```python
from build123d import *

# Parameters (mm, degrees)
SKETCH1_W           = 30
SKETCH1_H           = 120
BOSS_EXTRUDE1_DEPTH = 39
SKETCH2_OUTSIDE_W   = 57.94
SKETCH2_OUTSIDE_H   = 147.94
CUT_EXTRUDE2_DEPTH  = 74.116345642
FILLET1_R           = 5
CUT_EXTRUDE3_DEPTH  = 74.116345642
SKETCH4_W           = 4
SKETCH4_H           = 90
CUT_EXTRUDE4_DEPTH  = 72.902712049
SKETCH5_R           = 2
CUT_EXTRUDE5_DEPTH  = 72.902712049


with BuildPart() as part:
    # Sketch1 → Boss-Extrude1 (new body)
    with BuildSketch(Plane(origin=(0, 0, 0), x_dir=(1, 0, 0), z_dir=(0, 1, 0))):
        Rectangle(SKETCH1_W, SKETCH1_H)
    extrude(amount=BOSS_EXTRUDE1_DEPTH)

    # Sketch2 outside → Cut-Extrude2 (cut, through all)
    with BuildSketch(Plane(origin=(0, 39, 0), x_dir=(1, 0, 0), z_dir=(0, 1, 0))):
        Rectangle(SKETCH2_OUTSIDE_W, SKETCH2_OUTSIDE_H)
        Polygon((0, 60), (-15, 34.019237886), (-15, -60), (15, -60), (15, 34.019237886), align=None, mode=Mode.SUBTRACT)
    extrude(amount=-CUT_EXTRUDE2_DEPTH, mode=Mode.SUBTRACT)

    # Fillet1
    fillet1_edges = [part.edges().sort_by_distance(p)[0] for p in [
        (0, 19.5, -60),
    ]]
    fillet(fillet1_edges, radius=FILLET1_R)

    # Sketch3 → Cut-Extrude3 (cut, through all)
    with BuildSketch(Plane(origin=(0, 39, 0), x_dir=(1, 0, 0), z_dir=(0, 1, 0))):
        Polygon((-15, 34.019237886), (-15, -60), (-7, -60), (-7, 47.875644347), align=None)
        Polygon((7, 47.875644347), (7, -60), (15, -60), (15, 34.019237886), align=None)
    extrude(amount=-CUT_EXTRUDE3_DEPTH, mode=Mode.SUBTRACT)

    # Sketch4 → Cut-Extrude4 (cut, through all)
    with BuildSketch(Plane(origin=(0, 39, 0), x_dir=(1, 0, 0), z_dir=(0, 1, 0))):
        with Locations((-5, -15)):
            Rectangle(SKETCH4_W, SKETCH4_H)
    extrude(amount=-CUT_EXTRUDE4_DEPTH, mode=Mode.SUBTRACT)

    # Sketch5 → Cut-Extrude5 (cut, through all)
    with BuildSketch(Plane(origin=(0, 39, 0), x_dir=(1, 0, 0), z_dir=(0, 1, 0))):
        with Locations(Location((0, 46, 0), (0, 0, 270))):
            Circle(SKETCH5_R)
    extrude(amount=-CUT_EXTRUDE5_DEPTH, mode=Mode.SUBTRACT)


solid = part.part
```
Read the model definition and answer for the solid it produces. Units are mm, in the model's axes. A direction names the side the tool comes from. Coordinates: 2 decimals unless noted, no trailing zeros. Order: outer loops, then holes, each group sorted by start corner. A loop starts at its lowest first (then second) coordinate and runs counter-clockwise, first axis right, second up. Notation, with made-up numbers: (16.5, -1) - (68.5, -1) arc R29 ccw to (68.5, 29) - close; hole circle Ø7 at (69.25, -32). An arc over 180 degrees is marked (long way). Answer as a JSON object with one key per item and string values. Group by question number.
Item 1: Section C-C (z = 20) is taken. Give the vertices of the cut face in (x, y), plus the area to 3 significant figures.
Item 2: Section D-D (x = 6) is taken. Give the vertices of the cut face in (y, z), plus the area to 3 significant figures.
Item 3: The mould has two halves that part along Z. Classify faces 1 (the face through (-7, 20, -39)), 2 (the face through (5.68, 19.77, -50.16)), 3 (the face through (0, 20, -48)), 4 (the face through (2, 19, 60)): +Z half, -Z half, draft (parallel to the pull), parting line (faces both ways), or undercut.
Item 4: Flat-ended cylindrical pins translate along their axes: P1, Ø6, axis at x = -4.5, z = 34.5, coming from the -Y side; P2, Ø11.5, axis at y = 22, z = -7, coming from the -X side; P3, Ø1, axis at x = -5, y = 31.5, coming from the -Z side; P4, Ø4, axis at x = -3, y = 12, coming from the -Z side. Find the tip coordinate at first contact, or state that the pin passes through.
Item 5: A tool of negligible diameter and unlimited length cuts with its end or side. For faces 5 (the face through (-3, 20, 16)), 6 (the face through (0, 19, -55)), from which of +Z, -Z, +X, -X, +Y, -Y can it reach the whole face along a straight path? Write none if from no direction.
Item 6: Section A-A (z = -46) is taken. Give the vertices of the cut face in (x, y).
Item 7: Section B-B (y = 19) is taken. Give the vertices of the cut face in (x, z).
Item 8: Consider probe 1 along X at (y, z) = (26, -46); probe 2 along X at (y, z) = (27.5, 25); probe 3 along Z at (x, y) = (1.75, 32). Determine where each line is inside the solid, lowest interval first. Write a range as from..to.
Results are:
{
 "1": {"outline": "(-3, 0) - (7, 0) - (7, 39) - (-3, 39) - close", "area": "390 mm^2"},
 "2": {"outline": "(0, -49.61) - (39, -49.61) - (39, 60) - (0, 60) - close", "area": "4,270 mm^2"},
 "3": {"face 1": "draft", "face 2": "-Z half", "face 3": "undercut", "face 4": "+Z half"},
 "4": {"P1": "stops at y = 0", "P2": "stops at x = -3", "P3": "stops at z = -52.21", "P4": "stops at z = -54.9"},
 "5": {"face 5": "+Z, -X, +Y, -Y", "face 6": "-Z, +Y, -Y"},
 "6": {"outline": "(-7, 0) - (-2, 0) - (-2, 39) - (-7, 39) - close; (2, 0) - (7, 0) - (7, 39) - (2, 39) - close"},
 "7": {"outline": "(-7, -47.88) - (-4.33, -52.5) arc R5 ccw to (4.33, -52.5) - (7, -47.88) - (7, 60) - (-3, 60) - (-3, -30) - (-7, -30) - close; hole circle Ø4 at (0, -46)"},
 "8": {"probe 1": "x = -7..-2, 2..7", "probe 2": "x = -3..7", "probe 3": "z = -54.68..-46.97, -45.03..60"}
}
